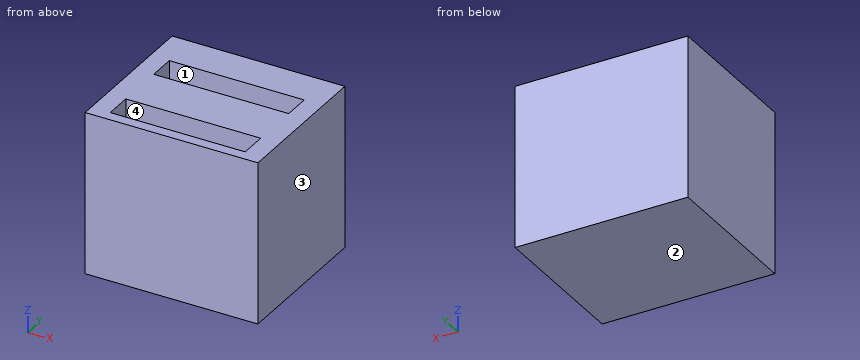
```python
from build123d import *

# Parameters (mm, degrees)
SKETCH1_W                                      = 640
SKETCH1_H                                      = 560
OVEN_OMAKE_FIRIN_SATIN_ALINAN_64X60X56_1_DEPTH = 600
OVEN_OMAKE_FIRIN_SATIN_ALINAN_64X60X56_2_START = 1
SKETCH2_W                                      = 500
SKETCH2_H                                      = 100
OVEN_OMAKE_FIRIN_SATIN_ALINAN_64X60X56_2_DEPTH = 421
OVEN_OMAKE_FIRIN_SATIN_ALINAN_64X60X56_3_START = 1
SKETCH3_W                                      = 500
SKETCH3_H                                      = 100
OVEN_OMAKE_FIRIN_SATIN_ALINAN_64X60X56_3_DEPTH = 421


with BuildPart() as part:
    # Sketch1 → OVEN_OMAKE_firin_SATIN_ALINAN_64x60x56_1 (new body)
    with BuildSketch(Plane.XY):
        with Locations((350, 1400)):
            Rectangle(SKETCH1_W, SKETCH1_H)
    extrude(amount=-OVEN_OMAKE_FIRIN_SATIN_ALINAN_64X60X56_1_DEPTH)

    # Sketch2 → OVEN_OMAKE_firin_SATIN_ALINAN_64x60x56_2 (cut)
    with BuildSketch(Plane.XY.offset(OVEN_OMAKE_FIRIN_SATIN_ALINAN_64X60X56_2_START)):
        with Locations((350, 1210)):
            Rectangle(SKETCH2_W, SKETCH2_H)
    extrude(amount=-OVEN_OMAKE_FIRIN_SATIN_ALINAN_64X60X56_2_DEPTH, mode=Mode.SUBTRACT)

    # Sketch3 → OVEN_OMAKE_firin_SATIN_ALINAN_64x60x56_3 (cut)
    with BuildSketch(Plane.XY.offset(OVEN_OMAKE_FIRIN_SATIN_ALINAN_64X60X56_3_START)):
        with Locations((350, 1490)):
            Rectangle(SKETCH3_W, SKETCH3_H)
    extrude(amount=-OVEN_OMAKE_FIRIN_SATIN_ALINAN_64X60X56_3_DEPTH, mode=Mode.SUBTRACT)


solid = part.part
```
Geometry: final body of the model. Coordinates: model frame, mm. Face numbers are marked on the shaded views. Round coordinates to 2 decimals unless told otherwise and drop trailing zeros. Order: outer loops, then holes, each group sorted by start corner. A loop starts at its lowest first (then second) coordinate and runs counter-clockwise, first axis right, second up. Notation, with made-up numbers: (82, -31) -> (139, -31) arc R18 cw to (139, 4) -> close; hole circle Ø1 at (81, -9.5). An arc over 180 degrees is marked (long way). Use CSV: the item, a comma, the result in double quotes. Start each with the question number.
1) Material intervals for line 1 along Y through (x, z) = (348, -188.5); line 2 along X through (y, z) = (1464, -28); line 3 along Z through (x, y) = (539, 1488), sorted ascending. Write a range as from..to.
2) Section C-C (z = -272). Return the cut outline in (x, y), and give its area (3 significant figures).
3) Section A-A (x = 307.5). Return the cut outline in (y, z).
4) Draft query along X for the marked faces 1, 2, 3 and 4. Return one class per face: +X half, -X half, draft (parallel to the pull), parting line (faces both ways), or undercut.
5) Section B-B (y = 1525.5). Return the cut outline in (x, z), and give its area (3 significant figures).
Returned:
1,line 1,"y = 1120..1160, 1260..1440, 1540..1680"
1,line 2,"x = 30..100, 600..670"
1,line 3,"z = -600..-420"
2,outline,"(30, 1120) -> (670, 1120) -> (670, 1680) -> (30, 1680) -> close; hole (100, 1160) -> (600, 1160) -> (600, 1260) -> (100, 1260) -> close; hole (100, 1440) -> (600, 1440) -> (600, 1540) -> (100, 1540) -> close"
2,area,"258,000 mm²"
3,outline,"(1120, -600) -> (1680, -600) -> (1680, 0) -> (1540, 0) -> (1540, -420) -> (1440, -420) -> (1440, 0) -> (1260, 0) -> (1260, -420) -> (1160, -420) -> (1160, 0) -> (1120, 0) -> close"
4,face 1,"undercut"
4,face 2,"draft"
4,face 3,"+X half"
4,face 4,"undercut"
5,outline,"(30, -600) -> (670, -600) -> (670, 0) -> (600, 0) -> (600, -420) -> (100, -420) -> (100, 0) -> (30, 0) -> close"
5,area,"174,000 mm²"
